```python
from build123d import *

# Parameters (mm, degrees)
BOSS_EXTRU_1_DEPTH      = 20
BOSS_EXTRU_2_START      = -20
BOSS_EXTRU_2_DEPTH      = 20
ESQUISSE3_R             = 1.65
ENL_V_MAT_EXTRU_1_DEPTH = 38.094473982
CONG_1_R                = 2


with BuildPart() as part:
    # Esquisse1 → Boss.-Extru.1 (new body)
    with BuildSketch(Plane.XY):
        with BuildLine():
            Line((6.739828673, -9.928479715), (14, -5))
            Line((14, -5), (14, 1.5))
            Line((14, 1.5), (9.886859967, 1.5))
            ThreePointArc((9.886859967, 1.5), (-9.742038622, -2.256697475), (9.539392014, 3))
            Line((9.539392014, 3), (14, 3))
            Line((14, 3), (14, 5))
            Line((14, 5), (6.739828673, 9.928479715))
            ThreePointArc((6.739828673, 9.928479715), (-12, 0), (6.739828673, -9.928479715))
        make_face()
    extrude(amount=BOSS_EXTRU_1_DEPTH)

    # Esquisse2 → Boss.-Extru.2 (add)
    with BuildSketch(Plane.XY.offset(20).offset(BOSS_EXTRU_2_START)):
        with BuildLine():
            Line((0, 12), (-20, 12))
            Line((-20, 12), (-20, 7))
            Line((-20, 7), (-9.681507645, -7.090021842))
            ThreePointArc((-9.681507645, -7.090021842), (-10.702342316, 5.427694625), (0, 12))
        make_face()
    extrude(amount=BOSS_EXTRU_2_DEPTH)

    # Esquisse3 → Enlèv. mat.-Extru.1 (cut, through all)
    with BuildSketch(Plane(origin=(0, 12, 0), x_dir=(1, 0, 0), z_dir=(0, 1, 0))):
        with Locations(Location((-15, -5, 0), (0, 0, 180))):
            Circle(ESQUISSE3_R)
        with Locations(Location((-15, -15, 0), (0, 0, 180))):
            Circle(ESQUISSE3_R)
    extrude(amount=-ENL_V_MAT_EXTRU_1_DEPTH, mode=Mode.SUBTRACT)

    # Congé1
    cong_1_edges = [part.edges().sort_by_distance(p)[0] for p in [
        (-20, 9.5, 0),
        (-20, 9.5, 20),
    ]]
    fillet(cong_1_edges, radius=CONG_1_R)


solid = part.part
```
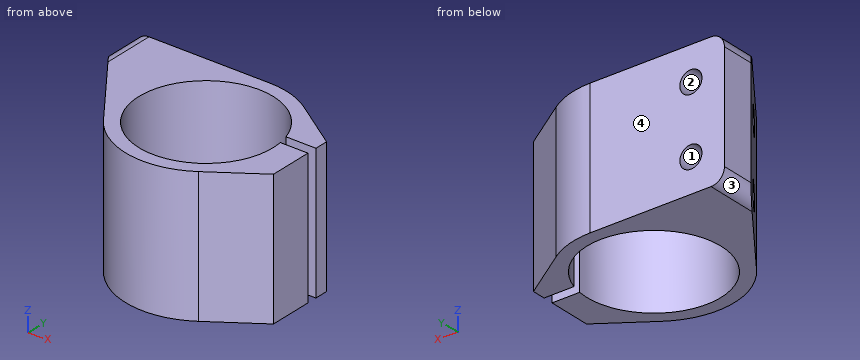
Work out the finished part from the listing and answer in its coordinate system (mm). Face numbers are marked on the shaded views. Give positions to 0.01 mm unless a question says otherwise; leave off trailing zeros. Write each loop counter-clockwise with the first axis right and the second up, starting at its lowest first coordinate (ties: lowest second). Pieces come first, ordered by that corner, then holes.
(1) The part is cut by section A-A on y = 9. Write down the section's boundary in (x, z).
Final values:
outline: (-20, 2) arc R2 ccw to (-18, 0) - (-4.36, 0) - (-4.36, 20) - (-18, 20) arc R2 ccw to (-20, 18) - close; (4.36, 0) - (8.11, 0) - (8.11, 20) - (4.36, 20) - close; hole circle Ø3.3 at (-15, 5); hole circle Ø3.3 at (-15, 15)
(2) Straight lines are drawn through the part: line 1 (Z direction, x = -15, y = 1); line 2 (X direction, y = 7.5, z = 5.5); line 3 (X direction, y = 3.5, z = 15). For each, find the intervals that lie inside material, in ascending order.
Final values:
line 1: z = 0 to 3.35, 6.65 to 13.35, 16.65 to 20
line 2: x = -20 to -16.57, -13.43 to -6.61, 6.61 to 10.32
line 3: x = -17.44 to -16.65, -13.35 to -9.37, 9.37 to 14
(3) The part is cut by section D-D on x = 4.5. Write down the section's boundary in (y, z), plus the area to 3 significant figures.
Final values:
outline: (-11.12, 0) - (-8.93, 0) - (-8.93, 20) - (-11.12, 20) - close; (8.93, 0) - (11.12, 0) - (11.12, 20) - (8.93, 20) - close
area: 87.8 mm2
(4) Flat-ended cylindrical pins translate along their axes: pin 1 Ø2 at (x, z) = (-15, 15) entering from +Y; pin 2 Ø3.5 at (x, z) = (11, 5.5) entering from -Y; pin 3 Ø3.5 at (x, z) = (12.5, 11.5) entering from +Y; pin 4 Ø3 at (y, z) = (1, 16.5) entering from -X. Find the tip coordinate at first contact, or state that the pin passes through.
Final values:
pin 1: passes through
pin 2: stops at y = -8.22
pin 3: stops at y = 7.21
pin 4: stops at x = -16.7
(5) The part is cut by section C-C on z = 8.25. Write down the section's boundary in (x, y).
Final values:
outline: (-20, 7) - (-9.68, -7.09) arc R12 ccw to (6.74, -9.93) - (14, -5) - (14, 1.5) - (9.89, 1.5) arc R10 cw (long way) to (9.54, 3) - (14, 3) - (14, 5) - (6.74, 9.93) arc R12 ccw to (0, 12) - (-20, 12) - close
(6) The mould has two halves that part along Z. Classify the marked faces 1, 2, 3 and 4: pulls with the +Z half, pulls with the -Z half, needs draft (parallel to the pull), parting line crosses it, or undercut.
Final values:
face 1: undercut
face 2: undercut
face 3: pulls with the -Z half
face 4: needs draft
(7) The part is cut by section B-B on z = 14. Write down the section's boundary in (x, y), plus the area to 3 significant figures.
Final values:
outline: (-20, 7) - (-16.31, 1.96) - (-16.31, 12) - (-20, 12) - close; (-13.69, -1.62) - (-9.68, -7.09) arc R12 ccw to (6.74, -9.93) - (14, -5) - (14, 1.5) - (9.89, 1.5) arc R10 cw (long way) to (9.54, 3) - (14, 3) - (14, 5) - (6.74, 9.93) arc R12 ccw to (0, 12) - (-13.69, 12) - close
area: 252 mm2
